For this review, use the dimensioned drawing (mm, ordinates from the lowest corner) and the shaded views. Coordinates: 2 decimals unless noted, no trailing zeros. Loops run counter-clockwise (first coordinate to the right, second up) from the corner with the lowest first, then second, coordinate; pieces in that order, holes last. Notation, with made-up numbers: M 38.5,-1 L 59.5,-1 A24 ccw 59.5,10 Z; hole C 75.5,86 d8. An arc over 180 degrees is marked long. Write item = value, one per line.
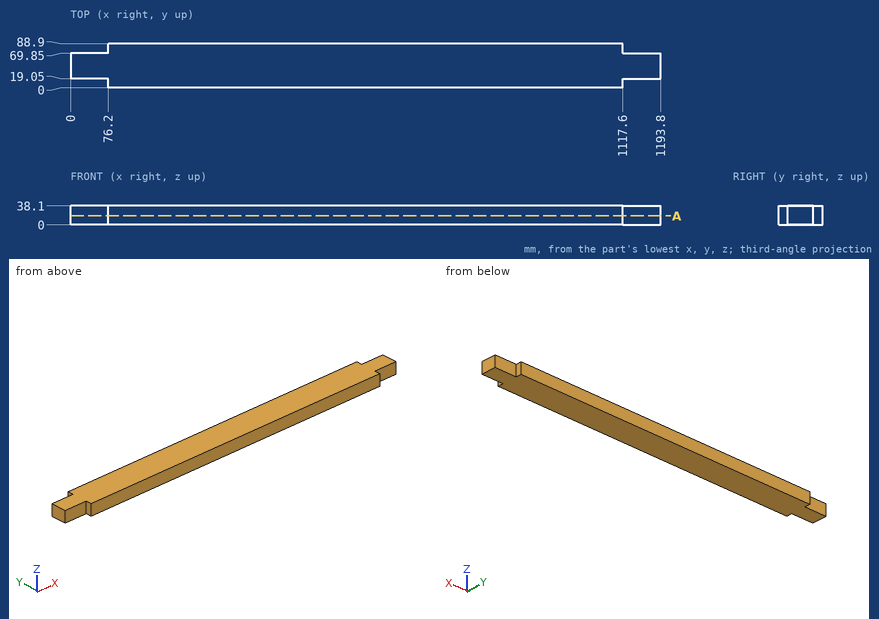
Q1. For pin 1 Ø3 at (y, z) = (77, 14) entering from +X; pin 2 Ø5.5 at (y, z) = (82, 11) entering from -X; pin 3 Ø11.5 at (x, z) = (1147, 11.5) entering from +Y, all flat-tipped, find the tip position at first contact; note any pin that passes through.
Solved:
pin_1 = 1117.6
pin_2 = 76.2
pin_3 = 69.85
Q2. For line 1 along X through (y, z) = (77, 14), list the stretches that pass through material, from the lowest coordinate up.
Solved:
line_1 = 76.2 to 1117.6
Q3. Add section A-A (z = 18). Write out the cut boundary in (x, y), and give its area (3 significant figures).
Solved:
outline = M 0,19.05 L 76.2,19.05 L 76.2,0 L 1117.6,0 L 1117.6,19.05 L 1193.8,19.05 L 1193.8,69.85 L 1117.6,69.85 L 1117.6,88.9 L 76.2,88.9 L 76.2,69.85 L 0,69.85 Z
area = 100,000 mm²
